CAD build for the part. Positions are in the model's coordinates, mm. A direction names the side the tool comes from. Give positions to 0.01 mm unless a question says otherwise; leave off trailing zeros. Loops run counter-clockwise (first coordinate to the right, second up) from the corner with the lowest first, then second, coordinate; pieces in that order, holes last.
```python
from build123d import *

# Parameters (mm, degrees)
F1_DEPTH = 30
F2_DEPTH = 2


with BuildPart() as f1:
    # F0 (on Top) → F1 (new body)
    with BuildSketch(Plane.XY):
        with BuildLine():
            Line((6.324367, 0.4), (14.318781, 0.4))
            ThreePointArc((14.318781, 0.4), (-14.324367, 0), (14.318781, -0.4))
            Line((14.318781, -0.4), (6.324367, -0.4))
            Line((6.324367, -0.4), (6.324367, 0.4))
        make_face()
    extrude(amount=F1_DEPTH)

    # F0 (on Top) → F2 (join)
    with BuildSketch(Plane.XY):
        with BuildLine():
            ThreePointArc((14.318781, -0.4), (-14.324367, 0), (14.318781, 0.4))
            Line((14.318781, 0.4), (16.319466, 0.4))
            ThreePointArc((16.319466, 0.4), (-16.324367, 0), (16.319466, -0.4))
            Line((16.319466, -0.4), (14.318781, -0.4))
        make_face()
        with BuildLine():
            Line((6.324367, 0.4), (14.318781, 0.4))
            ThreePointArc((14.318781, 0.4), (-14.324367, 0), (14.318781, -0.4))
            Line((14.318781, -0.4), (6.324367, -0.4))
            Line((6.324367, -0.4), (6.324367, 0.4))
        make_face()
    extrude(amount=-F2_DEPTH)


solid = f1.part
```
1. Tool access for faces 1 (the face through (0, 0, 30)), 2 (the face through (-1.29, -14.43, 0)): list every direction of +Z, -Z, +X, -X, +Y, -Y with a clear straight run to the whole face (end or side of a thin tool).
Responses:
face 1: +Z, +X, -X, +Y, -Y
face 2: +Z
2. Saw through at D-D, the plane z = 16. List the corners of the cut face in (x, y), and give its area (3 significant figures).
Responses:
outline: (6.32, -0.4) - (6.32, 0.4) - (14.32, 0.4) arc R14.32 ccw (long way) to (14.32, -0.4) - close
area: 638 mm2
3. Saw through at B-B, the plane y = -1. List the corners of the cut face in (x, z).
Responses:
outline: (-16.29, -2) - (16.29, -2) - (16.29, 0) - (14.29, 0) - (14.29, 30) - (-14.29, 30) - (-14.29, 0) - (-16.29, 0) - close
4. Drop flat-ended pins along their axis: pin 1 (1 mm diameter, centred on y = -9, z = 7, fed in from +X); pin 2 (1 mm diameter, centred on y = 8, z = 6, fed in from -X); pin 3 (11 mm diameter, centred on x = 11, z = 14, fed in from +Y). Give the stop position or say it passes through.
Responses:
pin 1: stops at x = 11.53
pin 2: stops at x = -12.2
pin 3: stops at y = 13.23
5. Saw through at A-A, the plane x = 0. List the corners of the cut face in (y, z), and give its area (3 significant figures).
Responses:
outline: (-16.32, -2) - (16.32, -2) - (16.32, 0) - (14.32, 0) - (14.32, 30) - (-14.32, 30) - (-14.32, 0) - (-16.32, 0) - close
area: 925 mm2
6. Saw through at C-C, the plane x = 8.5. List the corners of the cut face in (y, z), and give its area (3 significant figures).
Responses:
outline: (-13.94, -2) - (-0.4, -2) - (-0.4, 30) - (-11.53, 30) - (-11.53, 0) - (-13.94, 0) - close; (0.4, -2) - (13.94, -2) - (13.94, 0) - (11.53, 0) - (11.53, 30) - (0.4, 30) - close
area: 722 mm2
7. Probe line 1 along Y through (x, z) = (-0.5, 4); line 2 along Y through (x, z) = (9, 15); line 3 along Z through (x, y) = (6.5, 13). List the from-to ranges inside material, lowest first.
Responses:
line 1: y = -14.32 to 14.32
line 2: y = -11.14 to -0.4, 0.4 to 11.14
line 3: z = -2 to 0
8. Pull direction Y, two halves, no side cores. Call faces 3 (the face through (10, 0.4, 14)), 4 (the face through (0, 0, -2)), 5 (the face through (10, -0.4, 14)), 6 (the face through (-16.31, 0.71, -0.99)): released by +Y, released by -Y, zero draft, split by the parting line, or undercut.
Responses:
face 3: undercut
face 4: zero draft
face 5: undercut
face 6: split by the parting line
